The listing builds one solid part. Answer for the finished solid, in the listing's coordinates (mm). A direction names the side the tool comes from. Give positions to 0.01 mm unless a question says otherwise; leave off trailing zeros. Write each loop counter-clockwise with the first axis right and the second up, starting at its lowest first coordinate (ties: lowest second). Pieces come first, ordered by that corner, then holes.
```python
from build123d import *

# Parameters (mm, degrees)
SKETCH1_R           = 2.95
SKETCH1_R_2         = 2.2
BOSS_EXTRUDE1_DEPTH = 9
SKETCH2_R           = 10
BOSS_EXTRUDE2_DEPTH = 9


with BuildPart() as part:
    # Sketch1 → Boss-Extrude1 (new body)
    with BuildSketch(Plane(origin=(0, 0, 0), x_dir=(1, 0, 0), z_dir=(0, 1, 0))):
        Circle(SKETCH1_R)
        Circle(SKETCH1_R_2, mode=Mode.SUBTRACT)
    extrude(amount=BOSS_EXTRUDE1_DEPTH)

    # Sketch2 → Boss-Extrude2 (add)
    with BuildSketch(Plane(origin=(0, 9, 0), x_dir=(1, 0, 0), z_dir=(0, 1, 0))):
        Circle(SKETCH2_R)
    extrude(amount=BOSS_EXTRUDE2_DEPTH)


solid = part.part
```
Item 1: Determine the mould class of faces 3 (the face through (2.1, 4.44, -0.66)), 4 (the face through (2.1, 9, -2.4)), 5 (the face through (-2.947, 4.437, -0.13)) for opening direction Z: pulls with the +Z half, pulls with the -Z half, needs draft (parallel to the pull), parting line crosses it, or undercut.
Conclusion:
face 3: undercut
face 4: needs draft
face 5: parting line crosses it
Item 2: A cutting plane is placed at B-B, the plane y = 6.25. Give the vertices of the cut face in (x, z).
Conclusion:
outline: circle Ø5.9 at (0, 0); hole circle Ø4.4 at (0, 0)
Item 3: A cutting plane is placed at D-D, the plane y = 15.5. Give the vertices of the cut face in (x, z).
Conclusion:
outline: circle Ø20 at (0, 0)
Item 4: Consider probe 1 along X at (y, z) = (4.5, 0); probe 2 along Y at (x, z) = (-2, -7.5). Determine where each line is inside the solid, lowest interval first.
Conclusion:
probe 1: x = -2.95 to -2.2, 2.2 to 2.95
probe 2: y = 9 to 18
Item 5: A cutting plane is placed at A-A, the plane x = 0. Give the vertices of the cut face in (y, z).
Conclusion:
outline: (0, -2.95) - (9, -2.95) - (9, -10) - (18, -10) - (18, 10) - (9, 10) - (9, 2.95) - (0, 2.95) - (0, 2.2) - (9, 2.2) - (9, -2.2) - (0, -2.2) - close
Item 6: Which of the six approach directions +Z, -Z, +X, -X, +Y, -Y give full straight-line access (tool end or side, diameter ignored) to faces 1 (the face through (0, 18, 0)), 2 (the face through (0, 9, 0))?
Conclusion:
face 1: +Z, -Z, +X, -X, +Y
face 2: -Y
Item 7: Each of these flat-tipped pins is pushed along its axis until it touches: P1, Ø2, axis at x = -3.5, y = 5.5, coming from the -Z side; P2, Ø3, axis at y = 3.5, z = -0.5, coming from the +X side; P3, Ø1, axis at x = 4, y = 7, coming from the -Z side; P4, Ø1.5, axis at y = 9.5, z = 3, coming from the +X side. Where does it stop, or does it pass through?
Conclusion:
P1: stops at z = -1.57
P2: stops at x = 2.95
P3: passes through
P4: stops at x = 9.74
Item 8: A cutting plane is placed at C-C, the plane z = 0. Give the vertices of the cut face in (x, y).
Conclusion:
outline: (-10, 9) - (-2.95, 9) - (-2.95, 0) - (-2.2, 0) - (-2.2, 9) - (2.2, 9) - (2.2, 0) - (2.95, 0) - (2.95, 9) - (10, 9) - (10, 18) - (-10, 18) - close
